Geometry: see drawing. Coordinates: mm, zero at the bounding-box minimum. Coordinates: 2 decimals unless noted, no trailing zeros. Order: outer loops, then holes, each group sorted by start corner. A loop starts at its lowest first (then second) coordinate and runs counter-clockwise, first axis right, second up. Notation, with made-up numbers: (17.5, 53.25) - (35.5, 53.25) arc R25 ccw to (35.5, 85.25) - close; hole circle Ø10 at (-27.75, -17). An arc over 180 degrees is marked (long way). Use a Markdown table: item, result. Add a question column.
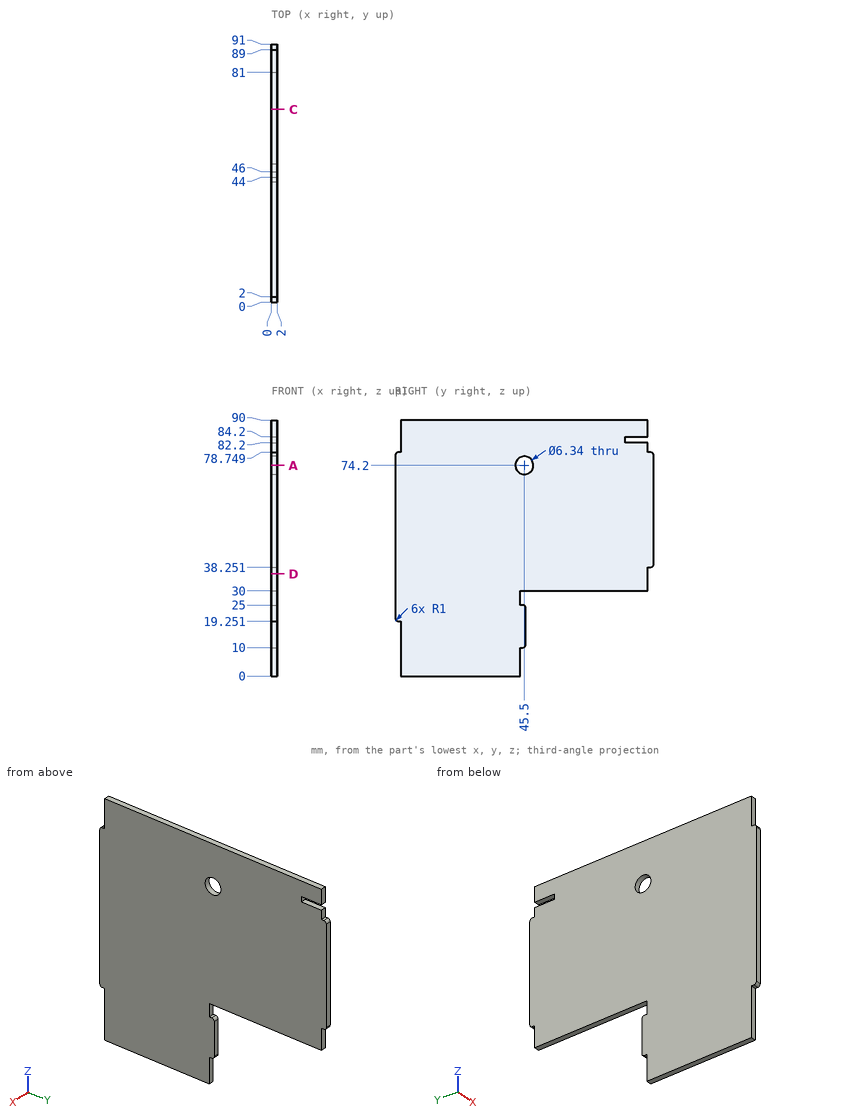
1) Section query D-D (z = 36). Return the cut outline in (x, y), and give its area (3 significant figures).
2) Section query A-A (z = 74.2). Return the cut outline in (x, y).
3) Section query C-C (y = 68). Return the cut outline in (x, z), and give its area (3 significant figures).
4) First-contact query: pin 1 (1 mm diameter, centred on x = 1, y = 83, fed in from -Z); pin 2 (1 mm diameter, centred on x = 1, z = 80.5, fed in from +Y); pin 3 (1 mm diameter, centred on x = 1, z = 19, fed in from +Y). Flat tips, straight axial feed; report the tip coordinate or a pass-through.
5) Line query: line 1 (Y direction, x = 0.5, z = 74.2); line 2 (Z direction, x = 1.45, y = 79.5); line 3 (Z direction, x = 1.05, y = 87). Output: solid intervals per line, ascending. Write a range as from..to.
From the geometry:
| question | item | result |
|---|---|---|
| 1 | outline | (0, 0) - (2, 0) - (2, 89) - (0, 89) - close |
| 1 | area | 178 mm^2 |
| 2 | outline | (0, 0) - (2, 0) - (2, 42.33) - (0, 42.33) - close; (0, 48.67) - (2, 48.67) - (2, 91) - (0, 91) - close |
| 3 | outline | (0, 30) - (2, 30) - (2, 90) - (0, 90) - close |
| 3 | area | 120 mm^2 |
| 4 | pin 1 | stops at z = 30 |
| 4 | pin 2 | stops at y = 89 |
| 4 | pin 3 | stops at y = 46 |
| 5 | line 1 | y = 0..42.33, 48.67..91 |
| 5 | line 2 | z = 30..90 |
| 5 | line 3 | z = 30..82.2, 84.2..90 |
